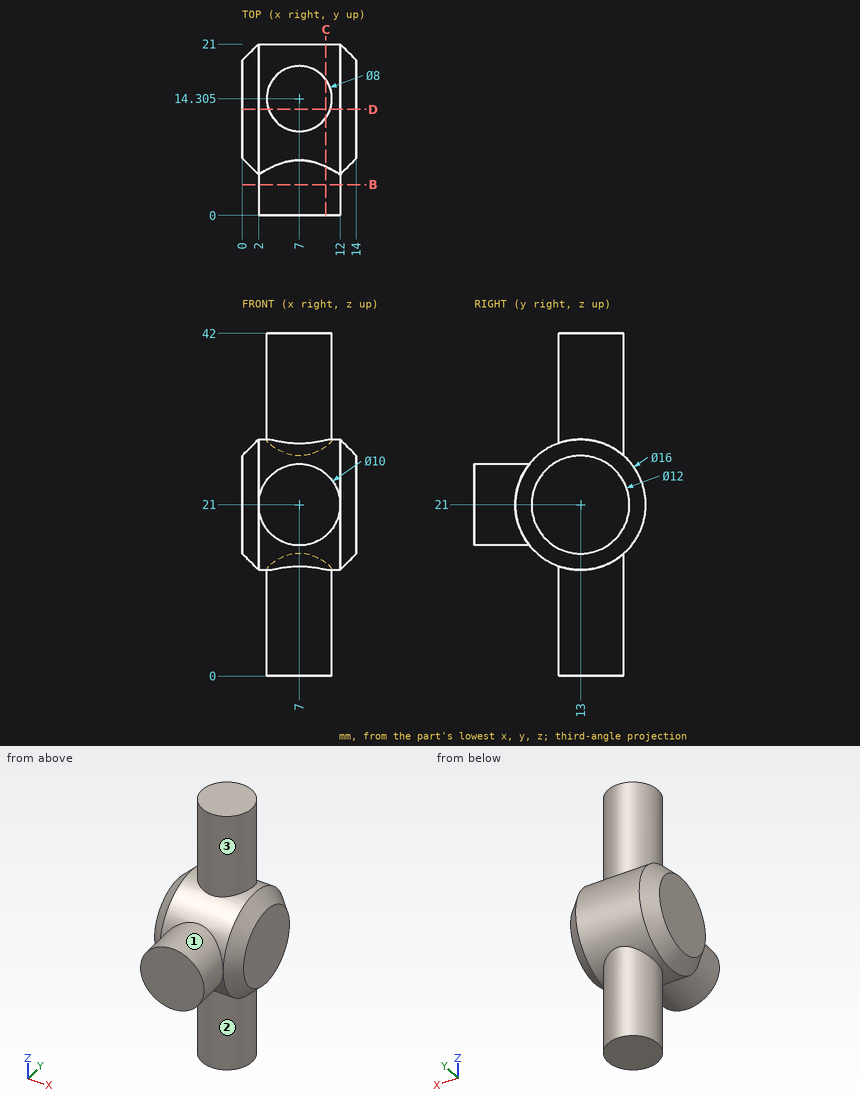
Design review of the part shown in the three views and the two pictorial views. Dimensions are in mm from the part's minimum x, y and z. A direction names the side the tool comes from. Give positions to 0.01 mm unless a question says otherwise; leave off trailing zeros. Order: outer loops, then holes, each group sorted by start corner. A loop starts at its lowest first (then second) coordinate and runs counter-clockwise, first axis right, second up. Notation, with made-up numbers: M 86,41 L 126,41 A14 cw 126,50 Z; hole C -33,39 d8. An arc over 180 degrees is marked long. Answer in a Markdown table with one row per item. Add a question column.
(1) Consider section B-B on y = 3.75. State the section outline as (x, z) points.
(2) For the marked faces 1, 2 and 3, list the 3-axis set-ups (+Z, -Z, +X, -X, +Y, -Y) from which the entire face can be reached by the end or side of a thin tool; tool diameter is ignored.
(3) Consider section C-C on x = 10.25. State the section outline as (y, z) points (1 decimal).
(4) For pin 1 (1.5 mm diameter, centred on y = 10, z = 31.5, fed in from +X) (1 decimal); pin 2 (3 mm diameter, centred on x = 1.5, z = 28, fed in from +Y); pin 3 (2 mm diameter, centred on x = 11.5, y = 19, fed in from -Z) (1 decimal), all flat-tipped, find the tip position at first contact; note any pin that passes through.
(5) Consider section D-D on y = 13. State the section outline as (x, z) points.
(6) Wall thickness on probe 1 along Y at (x, z) = (12.5, 27.5) (1 decimal); probe 2 along Z at (x, y) = (10, 10.5); probe 3 along Y at (x, z) = (7.5, 7): over which ranges is each line inside the solid? List them lowest first. Write a range as [from, to].
Evaluation:
| question | item | result |
|---|---|---|
| 1 | outline | C 7,21 d10 |
| 2 | face 1 | -Y |
| 2 | face 2 | -Z |
| 2 | face 3 | +Z |
| 3 | outline | M 0,17.2 L 6,17.2 A8 ccw 12,13.1 L 12,0 L 16.6,0 L 16.6,13.9 A8 ccw 16.6,28.1 L 16.6,42 L 12,42 L 12,28.9 A8 ccw 6,24.8 L 0,24.8 Z |
| 4 | pin 1 | stops at x = 8.8 |
| 4 | pin 2 | stops at y = 18.73 |
| 4 | pin 3 | stops at z = 14.8 |
| 5 | outline | M 0,15 L 2,13 L 3.22,13 L 3.22,0 L 10.78,0 L 10.78,13 L 12,13 L 14,15 L 14,27 L 12,29 L 10.78,29 L 10.78,42 L 3.22,42 L 3.22,29 L 2,29 L 0,27 Z |
| 6 | probe 1 | y = [9.3, 16.7] |
| 6 | probe 2 | z = [13.4, 28.6] |
| 6 | probe 3 | y = [10.34, 18.27] |
